Autodesk Inventor part; units mm, degrees
ref_plane "YZ Plane" through (0, 0, 0) normal (1, 0, 0) x (0, 1, 0)
ref_plane "XY Plane" through (0, 0, 0) normal (0, 0, 1) x (1, 0, 0)
sketch "Sketch3" plane through (0, 0, 0) normal (0, 0, 1) x (1, 0, 0)
  line L0 (0, 0) -> (0, 30)
  line L1 (0, 30) -> (1, 0)
  line L2 (1, 0) -> (0, 0)
  dimension "d3" = 30
  dimension "d4" = 1
revolve "Revolution1" add sketch "Sketch3" angle 360 about axis through (0, 0, 0) along (0, 1, 0)
ref_plane "Work Plane1" through (0, 30, 0) normal (0, 1, 0) x (-1, 0, 0)
sketch "Sketch5" plane through (0, 30, 0) normal (0, 1, 0) x (-1, 0, 0)
  circle A0 centre (0, 0) radius 1
  circle A1 centre (0, 0) radius 2.811
extrude "Extrusion3" cut sketch "Sketch5" against normal blind 5 contours A0 | A1
sketch "Sketch6" plane through (0, 0, 0) normal (0, -1, 0) x (1, 0, 0)
  circle A0 centre (0, 0) radius 0.1667
  circle A1 centre (0, 0) radius 1
extrude "Extrusion4" add sketch "Sketch6" along normal blind 1.2 contours A0 | A1
properties part number "LaserBeamEntry2x"
Geometry check sheet. Reference: the model listing, model coordinates, mm. A direction names the side the tool comes from. Round coordinates to 2 decimals unless told otherwise and drop trailing zeros. Write each loop counter-clockwise with the first axis right and the second up, starting at its lowest first coordinate (ties: lowest second). Pieces come first, ordered by that corner, then holes. Notation, with made-up numbers: (11.25, -22.75) -> (20.25, -22.75) arc R15 cw to (20.25, -6.75) -> close; hole circle Ø7 at (-15.75, -33). An arc over 180 degrees is marked (long way). Put each result on its own line as item: value.
1) Cross-section at B-B, the plane y = 9.5. Enter the section's corners in (x, z), plus the area to 3 significant figures.
Recorded:
outline: circle Ø1.37 at (0, 0)
area: 1.47 mm2
2) Depth check by flat-ended pin: P1, Ø1, axis at y = 9.5, z = 0.5, coming from the +X side; P2, Ø1, axis at y = 13.5, z = 0, coming from the +X side. Enter the tip coordinate at first touch or a pass-through.
Recorded:
P1: stops at x = 0.69
P2: stops at x = 0.57
3) Cross-section at A-A, the plane y = 1.25. Enter the section's corners in (x, z), plus the area to 3 significant figures.
Recorded:
outline: circle Ø1.92 at (0, 0)
area: 2.89 mm2
4) Thickness scan on probe 1 along Z at (x, y) = (0.1, 2.5); probe 2 along X at (y, z) = (3.5, 0.7); probe 3 along X at (y, z) = (16, 0.3). Record the ranges inside material, lowest first. Write a range as from..to.
Recorded:
probe 1: z = -0.91..0.91
probe 2: x = -0.54..0.54
probe 3: x = -0.36..0.36
5) Access from +Z, -Z, +X, -X, +Y, -Y to the whole of each face (thin tool, end or side, straight path). Record for faces 1 (the face through (0, -1, 1)), 2 (the face through (0.56, 12.32, 0.18)).
Recorded:
face 1: +Y, -Y
face 2: +Y
